The listing builds one solid part. Answer for the finished solid, in the listing's coordinates (mm). Round coordinates to 2 decimals unless told otherwise and drop trailing zeros. Loops run counter-clockwise (first coordinate to the right, second up) from the corner with the lowest first, then second, coordinate; pieces in that order, holes last. Notation, with made-up numbers: M 5.25,24 L 20.25,24 A23 cw 20.25,49 Z; hole C 62,82.25 d8. An arc over 180 degrees is marked long. Put each result on its own line as item: value. Start each with the question number.
(1) Flat-ended cylindrical pins translate along their axes: P1, Ø3, axis at x = -64.35, y = 64.35, coming from the +Z side; P2, Ø1.5, axis at x = 71.5, z = -6.5, coming from the -Y side; P3, Ø4, axis at y = 45, z = -8, coming from the +X side; P4, Ø4, axis at y = 31.5, z = -9, coming from the +X side. Find the tip coordinate at first contact, or state that the pin passes through.
(2) Section D-D, the plane y = 51 is taken. Determine the outline of the cut face in (x, z), then the cut area to 3 significant figures.
(3) Determine the mould class of faces 1 (the face through (-23.412, 105.432, -4.93)), 2 (the face through (46, -2, 0)), 3 (the face through (-8.67, 39.05, -4.93)) for opening direction X: released by +X, released by -X, zero draft, split by the parting line, or undercut.
(4) Section B-B, the plane x = -22 is taken. Determine the outline of the cut face in (y, z), then the cut area to 3 significant figures.
(5) Straight lines are drawn through the part: line 1 (Y direction, x = 0, z = -3.75); line 2 (Y direction, x = -8.5, z = -4); line 3 (Y direction, x = 34, z = -4.5). For each, find the intervals that lie inside material, in ascending order.
(6) Section C-C, the plane z = -8 is taken. Count the separate pieces of the cut face and the enclosed holes in it, then the cut area to 3 significant figures.
(7) Section A-A, the plane y = -5.5 is taken. Determine the outline of the cut face in (x, z), then the cut area to 3 significant figures.
```python
from build123d import *

# Parameters (mm, degrees)
SKETCH001_R       = 108
SKETCH001_R_2     = 40
SKETCH001_R_3     = 2.5
SKETCH001_R_4     = 1.5625
PAD_DEPTH         = 10
SKETCH_R          = 1.5625
POCKET_DEPTH      = 10.001
POCKET_DEPTH_BACK = 0.001


with BuildPart() as part:
    # Sketch001 → Pad (new body)
    with BuildSketch(Plane(origin=(0, 0, 0), x_dir=(1, 0, 0), z_dir=(0, 0, -1))):
        Circle(SKETCH001_R)
        Circle(SKETCH001_R_2, mode=Mode.SUBTRACT)
        with Locations((38.651027, 93.311833)):
            Circle(SKETCH001_R_3, mode=Mode.SUBTRACT)
        with Locations((93.311833, 38.651027)):
            Circle(SKETCH001_R_3, mode=Mode.SUBTRACT)
        with Locations((93.311833, -38.651027)):
            Circle(SKETCH001_R_3, mode=Mode.SUBTRACT)
        with Locations((38.651027, -93.311833)):
            Circle(SKETCH001_R_3, mode=Mode.SUBTRACT)
        with Locations((-38.651027, 93.311833)):
            Circle(SKETCH001_R_3, mode=Mode.SUBTRACT)
        with Locations((-93.311833, 38.651027)):
            Circle(SKETCH001_R_3, mode=Mode.SUBTRACT)
        with Locations((-93.311833, -38.651027)):
            Circle(SKETCH001_R_3, mode=Mode.SUBTRACT)
        with Locations((-38.651027, -93.311833)):
            Circle(SKETCH001_R_3, mode=Mode.SUBTRACT)
        with Locations((0, 60)):
            Circle(SKETCH001_R_4, mode=Mode.SUBTRACT)
        with Locations((-60, 0)):
            Circle(SKETCH001_R_4, mode=Mode.SUBTRACT)
        with Locations((0, -60)):
            Circle(SKETCH001_R_4, mode=Mode.SUBTRACT)
        with Locations((60, 0)):
            Circle(SKETCH001_R_4, mode=Mode.SUBTRACT)
    extrude(amount=PAD_DEPTH)

    # Sketch → Pocket (cut, two sides)
    with BuildSketch(Plane.XY) as pocket_sk:
        with Locations((64.346717, 64.346717)):
            Circle(SKETCH_R)
        with Locations((0, 91)):
            Circle(SKETCH_R)
        with Locations((91, 0)):
            Circle(SKETCH_R)
        with Locations((64.346717, -64.346717)):
            Circle(SKETCH_R)
        with Locations((0, -91)):
            Circle(SKETCH_R)
        with Locations((-91, 0)):
            Circle(SKETCH_R)
        with Locations((-64.346717, -64.346717)):
            Circle(SKETCH_R)
        with Locations((-64.346717, 64.346717)):
            Circle(SKETCH_R)
    extrude(amount=-POCKET_DEPTH, mode=Mode.SUBTRACT)
    extrude(pocket_sk.sketch, amount=POCKET_DEPTH_BACK, mode=Mode.SUBTRACT)


solid = part.part
```
Recorded:
1. P1: passes through
1. P2: stops at y = -81.6
1. P3: stops at x = 99.07
1. P4: stops at x = 103.89
2. outline: M -95.2,-10 L 95.2,-10 L 95.2,0 L -95.2,0 Z
2. area: 1,900 mm²
3. face 1: split by the parting line
3. face 2: zero draft
3. face 3: undercut
4. outline: M -105.74,-10 L -33.41,-10 L -33.41,0 L -105.74,0 Z; M 33.41,-10 L 105.74,-10 L 105.74,0 L 33.41,0 Z
4. area: 1,450 mm²
5. line 1: y = -108 to -92.56, -89.44 to -61.56, -58.44 to -40, 40 to 58.44, 61.56 to 89.44, 92.56 to 108
5. line 2: y = -107.66 to -39.09, 39.09 to 107.66
5. line 3: y = -102.51 to -21.07, 21.07 to 102.51
6. separate pieces: 1
6. enclosed holes: 21
6. area: 31,400 mm²
7. outline: M -107.86,-10 L -39.62,-10 L -39.62,0 L -107.86,0 Z; M 39.62,-10 L 107.86,-10 L 107.86,0 L 39.62,0 Z
7. area: 1,360 mm²
